```python
from build123d import *

# Parameters (mm, degrees)
SKETCH1_W           = 63.5
SKETCH1_H           = 63.5
BOSS_EXTRUDE1_DEPTH = 152.4
SKETCH2_W           = 142.24
SKETCH2_H           = 53.34
CUT_EXTRUDE1_DEPTH  = 58.42
FILLET1_R           = 2
FILLET2_R           = 1.2
SCALE1_SCALE        = 0.06


with BuildPart() as part:
    # Sketch1 → Boss-Extrude1 (new body)
    with BuildSketch(Plane(origin=(0, 0, 0), x_dir=(0, 0, -1), z_dir=(1, 0, 0))):
        Rectangle(SKETCH1_W, SKETCH1_H)
    extrude(amount=BOSS_EXTRUDE1_DEPTH)

    # Sketch2 → Cut-Extrude1 (cut)
    with BuildSketch(Plane(origin=(0, 31.75, 0), x_dir=(1, 0, 0), z_dir=(0, 1, 0))):
        with Locations((76.2, 0)):
            Rectangle(SKETCH2_W, SKETCH2_H)
    extrude(amount=-CUT_EXTRUDE1_DEPTH, mode=Mode.SUBTRACT)

    # Fillet1
    fillet1_edges = [part.edges().sort_by_distance(p)[0] for p in [
        (152.4, 0, 31.75),
        (152.4, 0, -31.75),
        (0, 0, 31.75),
        (0, 0, -31.75),
    ]]
    fillet(fillet1_edges, radius=FILLET1_R)

    # Fillet2
    fillet2_edges = [part.edges().sort_by_distance(p)[0] for p in [
        (152.4, 31.75, 0),
        (76.2, 31.75, 31.75),
        (0, 31.75, 0),
        (76.2, 31.75, -31.75),
        (0.585786438, 31.75, 31.164213562),
        (0.585786438, 31.75, -31.164213562),
        (151.814213562, 31.75, -31.164213562),
        (151.814213562, 31.75, 31.164213562),
    ]]
    fillet(fillet2_edges, radius=FILLET2_R)


with BuildPart() as part_1:
    # Scale1: scaled about (76.2, -6.610828931, 0)
    add(part.part.scale(SCALE1_SCALE).moved(Location((71.628, -6.214179195, 0))))


solid = part_1.part
```
CAD build for the part. Positions are in the model's coordinates, mm. A direction names the side the tool comes from. Round coordinates to 2 decimals unless told otherwise and drop trailing zeros. Order: outer loops, then holes, each group sorted by start corner. A loop starts at its lowest first (then second) coordinate and runs counter-clockwise, first axis right, second up.
Q1. Two-plate mould, pull along Z, no slides. Class faces 1 (the flat face through (76, -8.119, 0)), 2 (the flat face through (76, -7.814, 0)), 3 (the flat face through (76, -6, -1.905)), 4 (the flat face through (71.933, -6, 0)): pulls with the +Z half, pulls with the -Z half, needs draft (parallel to the pull), parting line crosses it, or undercut.
Q2. Slice it at A-A (y = -7.35). Write the cut outline in (x, z) (3 decimals).
Q3. Slice it at B-B (z = 0). Write the cut outline in (x, y).
Q4. Which spindle directions (+Z, -Z, +X, -X, +Y, -Y) get a long thin tool onto all of the face, cutting with end or side? Do faces 5 (the flat face through (76, -6, -1.6)), 6 (the flat face through (76, -6, 1.905)). Say none if no direction does.
Q5. Slice it at C-C (x = 77). Write the cut outline in (y, z) (3 decimals).
Q6. Drop a flat-ended pin along its axis: pin 1 (1.6 mm diameter, centred on x = 74, z = 0, fed in from +Y). Give the stop position or say it passes through.
Q7. Wall check: L1, parallel to X at y = -7.2, z = -0.15; L2, parallel to Z at x = 77.5, y = -6.65 (3 decimals); L3, parallel to Y at x = 73.5, z = -1.35. Give the ranges that are in metal, low to high.
Results below:
1. face 1: needs draft
1. face 2: undercut
1. face 3: pulls with the -Z half
1. face 4: undercut
2. outline: (71.628, -1.785) arc R0.12 ccw to (71.748, -1.905) - (80.652, -1.905) arc R0.12 ccw to (80.772, -1.785) - (80.772, 1.785) arc R0.12 ccw to (80.652, 1.905) - (71.748, 1.905) arc R0.12 ccw to (71.628, 1.785) - close; hole (71.933, -1.6) - (80.467, -1.6) - (80.467, 1.6) - (71.933, 1.6) - close
3. outline: (71.63, -8.12) - (80.77, -8.12) - (80.77, -4.38) arc R0.07 ccw to (80.7, -4.31) - (80.47, -4.31) - (80.47, -7.81) - (71.93, -7.81) - (71.93, -4.31) - (71.7, -4.31) arc R0.07 ccw to (71.63, -4.38) - close
4. face 5: +Y
4. face 6: +Z, +X, -X, +Y, -Y
5. outline: (-8.119, -1.905) - (-4.381, -1.905) arc R0.072 ccw to (-4.309, -1.833) - (-4.309, -1.6) - (-7.814, -1.6) - (-7.814, 1.6) - (-4.309, 1.6) - (-4.309, 1.833) arc R0.072 ccw to (-4.381, 1.905) - (-8.119, 1.905) - close
6. pin 1: stops at y = -7.81
7. L1: x = 71.63 to 71.93, 80.47 to 80.77
7. L2: z = -1.905 to -1.6, 1.6 to 1.905
7. L3: y = -8.12 to -7.81
